```python
from build123d import *
from OCP.BRepFilletAPI import BRepFilletAPI_MakeChamfer

# Parameters (mm, degrees)
SKETCH1_R                      = 155
BOSS_EXTRUDE1_DEPTH            = 3.1
SKETCH2_R                      = 1.65
CUT_EXTRUDE1_DEPTH             = 220.225021382
SKETCH3_R                      = 3.25
CUT_EXTRUDE2_DEPTH             = 2
CHAMFER1_SIZE2                 = 1.6
CHAMFER1_SIZE                  = 1.1
CIRPATTERN1_COUNT              = 6
CHAMFER1_OF_CIRPATTERN1_SIZE   = 1.1
CHAMFER1_OF_CIRPATTERN1_SIZE_2 = 1.6
CUT_EXTRUDE3_DEPTH             = 220.225021382


with BuildPart() as part:
    # Sketch1 → Boss-Extrude1 (new body)
    with BuildSketch(Plane(origin=(0, 0, 0), x_dir=(1, 0, 0), z_dir=(0, 1, 0))):
        with Locations(Location((0, 0, 0), (0, 0, 90))):
            Circle(SKETCH1_R)
    extrude(amount=BOSS_EXTRUDE1_DEPTH)

    # Sketch2 → Cut-Extrude1 (cut, through all)
    with BuildSketch(Plane(origin=(0, 3.1, 0), x_dir=(1, 0, 0), z_dir=(0, 1, 0))):
        with Locations(Location((150, 0, 0), (0, 0, 270))):
            Circle(SKETCH2_R)
    cut_extrude1 = extrude(amount=-CUT_EXTRUDE1_DEPTH, mode=Mode.SUBTRACT)

    # Sketch3 → Cut-Extrude2 (cut)
    with BuildSketch(Plane(origin=(0, 3.1, 0), x_dir=(1, 0, 0), z_dir=(0, 1, 0))):
        with Locations(Location((150, 0, 0), (0, 0, 270))):
            Circle(SKETCH3_R)
    cut_extrude2 = extrude(amount=-CUT_EXTRUDE2_DEPTH, mode=Mode.SUBTRACT)

    # Chamfer1
    chamfer1_edges = [part.edges().sort_by_distance(p)[0] for p in [
        (150, 1.1, -1.65),
    ]]
    chamfer1_side = [part.faces().sort_by_distance(p)[0] for p in [
        (150, 1.078, -1.65),
    ]]
    chamfer(chamfer1_edges, length=CHAMFER1_SIZE - 0.0001, length2=CHAMFER1_SIZE2 - 0.0001, reference=chamfer1_side[0])  # a hair under: the kernel refuses the full size

    # CirPattern1: Cut-Extrude1, Cut-Extrude2 ×6 about axis
    cirpattern1_axis = Axis((0, 0, 0), (0, 1, 0))
    add([cut_extrude1.rotate(cirpattern1_axis, i * 360 / CIRPATTERN1_COUNT) for i in range(1, CIRPATTERN1_COUNT)], mode=Mode.SUBTRACT)
    add([cut_extrude2.rotate(cirpattern1_axis, i * 360 / CIRPATTERN1_COUNT) for i in range(1, CIRPATTERN1_COUNT)], mode=Mode.SUBTRACT)

    # Chamfer1 of CirPattern1
    chamfer1_of_cirpattern1_edges_1 = [part.edges().sort_by_distance(p)[0] for p in [
        (73.571058084, 1.1, -130.728810568),
    ]]
    chamfer1_of_cirpattern1_side_1 = [part.faces().sort_by_distance(p)[0] for p in [
        (73.571058084, 1.078, -130.728810568),
    ]]
    chamfer1_of_cirpattern1_edges_2 = [part.edges().sort_by_distance(p)[0] for p in [
        (-76.428941916, 1.1, -129.078810568),
    ]]
    chamfer1_of_cirpattern1_side_2 = [part.faces().sort_by_distance(p)[0] for p in [
        (-76.428941916, 1.078, -129.078810568),
    ]]
    chamfer1_of_cirpattern1_edges_3 = [part.edges().sort_by_distance(p)[0] for p in [
        (-150, 1.1, 1.65),
    ]]
    chamfer1_of_cirpattern1_side_3 = [part.faces().sort_by_distance(p)[0] for p in [
        (-150, 1.078, 1.65),
    ]]
    chamfer1_of_cirpattern1_edges_4 = [part.edges().sort_by_distance(p)[0] for p in [
        (-73.571058084, 1.1, 130.728810568),
    ]]
    chamfer1_of_cirpattern1_side_4 = [part.faces().sort_by_distance(p)[0] for p in [
        (-73.571058084, 1.078, 130.728810568),
    ]]
    chamfer1_of_cirpattern1_edges_5 = [part.edges().sort_by_distance(p)[0] for p in [
        (76.428941916, 1.1, 129.078810568),
    ]]
    chamfer1_of_cirpattern1_side_5 = [part.faces().sort_by_distance(p)[0] for p in [
        (76.428941916, 1.078, 129.078810568),
    ]]
    chamfer1_of_cirpattern1 = BRepFilletAPI_MakeChamfer(part.part.solid().wrapped)
    for e in chamfer1_of_cirpattern1_edges_1:
        chamfer1_of_cirpattern1.Add(CHAMFER1_OF_CIRPATTERN1_SIZE - 0.0001, CHAMFER1_OF_CIRPATTERN1_SIZE_2 - 0.0001, e.wrapped, chamfer1_of_cirpattern1_side_1[0].wrapped)
    for e in chamfer1_of_cirpattern1_edges_2:
        chamfer1_of_cirpattern1.Add(CHAMFER1_OF_CIRPATTERN1_SIZE - 0.0001, CHAMFER1_OF_CIRPATTERN1_SIZE_2 - 0.0001, e.wrapped, chamfer1_of_cirpattern1_side_2[0].wrapped)
    for e in chamfer1_of_cirpattern1_edges_3:
        chamfer1_of_cirpattern1.Add(CHAMFER1_OF_CIRPATTERN1_SIZE - 0.0001, CHAMFER1_OF_CIRPATTERN1_SIZE_2 - 0.0001, e.wrapped, chamfer1_of_cirpattern1_side_3[0].wrapped)
    for e in chamfer1_of_cirpattern1_edges_4:
        chamfer1_of_cirpattern1.Add(CHAMFER1_OF_CIRPATTERN1_SIZE - 0.0001, CHAMFER1_OF_CIRPATTERN1_SIZE_2 - 0.0001, e.wrapped, chamfer1_of_cirpattern1_side_4[0].wrapped)
    for e in chamfer1_of_cirpattern1_edges_5:
        chamfer1_of_cirpattern1.Add(CHAMFER1_OF_CIRPATTERN1_SIZE - 0.0001, CHAMFER1_OF_CIRPATTERN1_SIZE_2 - 0.0001, e.wrapped, chamfer1_of_cirpattern1_side_5[0].wrapped)
    add(Compound.cast(chamfer1_of_cirpattern1.Shape()), mode=Mode.REPLACE)  # a hair under: the kernel refuses the full size

    # Sketch4 → Cut-Extrude3 (cut, through all)
    with BuildSketch(Plane(origin=(0, 3.1, 0), x_dir=(1, 0, 0), z_dir=(0, 1, 0))):
        with BuildLine():
            Line((0, 150.013332741), (39, 150.013332741))
            ThreePointArc((39, 150.013332741), (0, 155), (-39, 150.013332741))
            Line((-39, 150.013332741), (0, 150.013332741))
        make_face()
    extrude(amount=-CUT_EXTRUDE3_DEPTH, mode=Mode.SUBTRACT)


solid = part.part
```
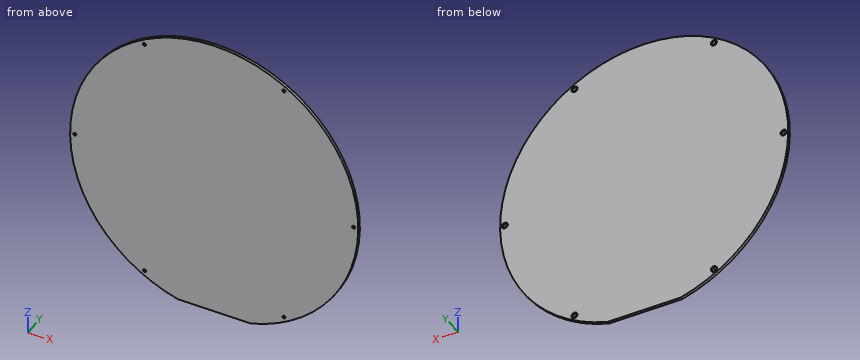
Check sheet for the modelled part. Datum: model origin and axes. Units: mm. Round coordinates to 2 decimals unless told otherwise and drop trailing zeros. Loops run counter-clockwise (first coordinate to the right, second up) from the corner with the lowest first, then second, coordinate; pieces in that order, holes last. Notation, with made-up numbers: M 81,59 L 96,59 A20 ccw 96,83 Z; hole C 54.25,17 d11. An arc over 180 degrees is marked long. Answer as a JSON object with one key per item and string values.
1. Section check A-A (y = 1.75). Record the boundary of the cut face in (x, z), plus the area to 3 significant figures.
Reply:
{"outline": "M -39,-150.01 L 39,-150.01 A155 ccw long Z; hole C -150,0 d6.5; hole C -75,-129.9 d6.5; hole C -75,129.9 d6.5; hole C 75,-129.9 d6.5; hole C 75,129.9 d6.5; hole C 150,0 d6.5", "area": "75,000 mm²"}
2. Section check C-C (z = -108). Record the boundary of the cut face in (x, y), plus the area to 3 significant figures.
Reply:
{"outline": "M -111.18,0 L 111.18,0 L 111.18,3.1 L -111.18,3.1 Z", "area": "689 mm²"}
3. Scan lines: line 1 (X direction, y = 0.05, z = 0); line 2 (X direction, y = 1.75, z = -129.5); line 3 (Z direction, x = -121.5, y = 1.2). Record each from-to range of solid material in increasing order.
Reply:
{"line 1": "x = -155 to -151.72, -148.28 to 148.28, 151.72 to 155", "line 2": "x = -85.17 to -78.22, -71.78 to 71.78, 78.22 to 85.17", "line 3": "z = -96.24 to 96.24"}
4. Section check B-B (x = 50.5). Record the boundary of the cut face in (y, z), plus the area to 3 significant figures.
Reply:
{"outline": "M 0,-146.54 L 3.1,-146.54 L 3.1,146.54 L 0,146.54 Z", "area": "909 mm²"}
5. Gauge pin test, flat ends, axial feed: P1, Ø3, axis at x = 75.5, z = 129.5, coming from the +Y side; P2, Ø3, axis at x = 75.5, z = -130.5, coming from the +Y side; P3, Ø6, axis at x = 75, z = 129.9, coming from the +Y side. Record the tip position at first contact, or that the pin passes through.
Reply:
{"P1": "stops at y = 0.34", "P2": "stops at y = 0.43", "P3": "stops at y = 0.93"}
